Answer from the drawing. Dimensions are ordinates in mm from the lowest x, y and z of the part. A direction names the side the tool comes from. Coordinates: 2 decimals unless noted, no trailing zeros. Order: outer loops, then holes, each group sorted by start corner. A loop starts at its lowest first (then second) coordinate and runs counter-clockwise, first axis right, second up.
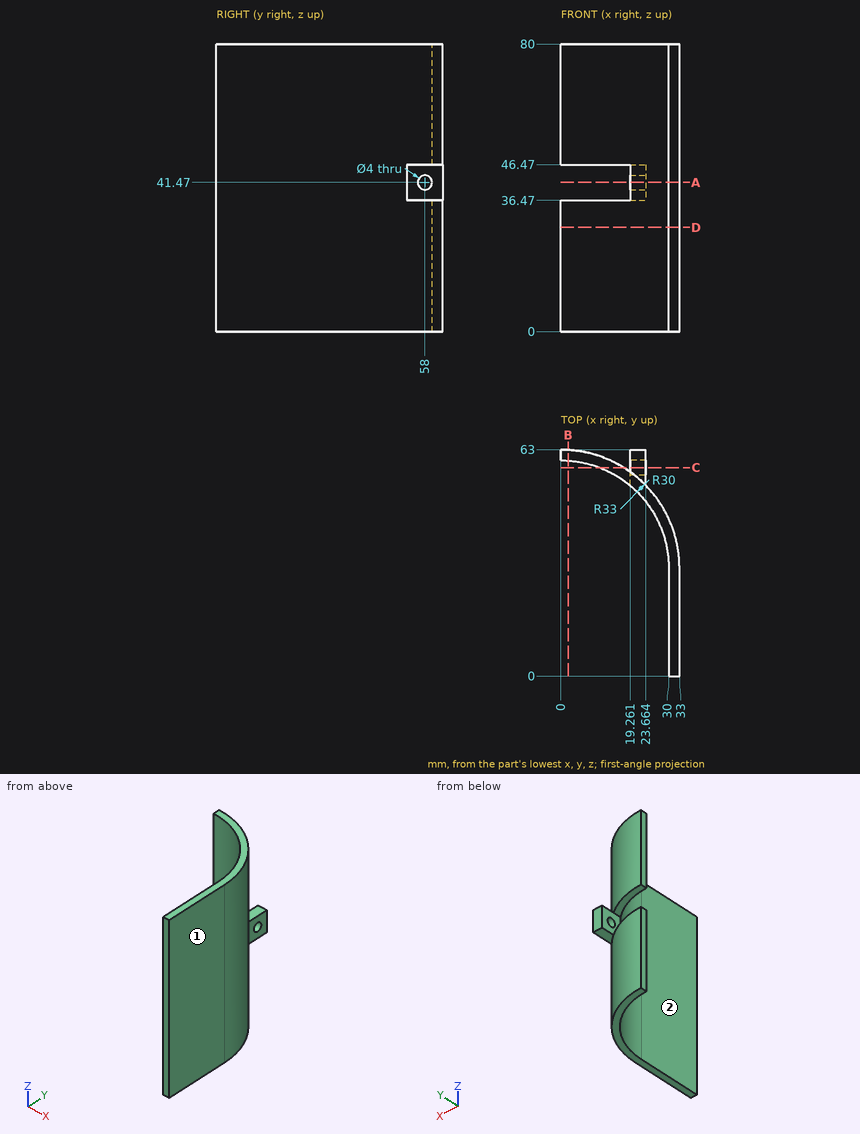
1. Flat-ended cylindrical pins translate along their axes: pin 1 (3 mm diameter, centred on y = 59, z = 39, fed in from -X); pin 2 (2 mm diameter, centred on x = 21, y = 60, fed in from +Z); pin 3 (15 mm diameter, centred on y = 16.5, z = 48, fed in from -X). Find the tip coordinate at first contact, or state that the pin passes through.
2. Consider probe 1 along Z at (x, y) = (21.85, 58); probe 2 along X at (y, z) = (14.5, 27.5); probe 3 along Y at (x, z) = (20, 41) (1 decimal). Determine where each line is inside the solid, lowest interval first.
3. The part is cut by section C-C (y = 58). Determine the outline of the cut face in (x, z) (1 decimal), plus the area to 3 significant figures.
4. The part is cut by section D-D (z = 29). Determine the outline of the cut face in (x, y).
5. The part is cut by section A-A (z = 41.47). Determine the outline of the cut face in (x, y) (1 decimal), plus the area to 3 significant figures.
6. For the marked faces 1 and 2, determine the directions among +Z, -Z, +X, -X, +Y, -Y from which every point of the face is accessible in a straight line to the end or side of a thin tool.
7. The part is cut by section B-B (x = 2). Determine the outline of the cut face in (y, z).
Worked out:
1. pin 1: stops at x = 19.26
1. pin 2: stops at z = 46.47
1. pin 3: stops at x = 30
2. probe 1: z = 36.47 to 39.47, 43.47 to 46.47
2. probe 2: x = 30 to 33
2. probe 3: y = 52.4 to 56.1, 59.9 to 63
3. outline: (10.8, 0) - (17.5, 0) - (17.5, 36.5) - (10.8, 36.5) - close; (10.8, 46.5) - (17.5, 46.5) - (17.5, 80) - (10.8, 80) - close; (19.3, 36.5) - (23.7, 36.5) - (23.7, 39.5) - (19.3, 39.5) - close; (19.3, 43.5) - (23.7, 43.5) - (23.7, 46.5) - (19.3, 46.5) - close
3. area: 495 mm2
4. outline: (0, 60) arc R30 cw to (30, 30) - (30, 0) - (33, 0) - (33, 30) arc R33 ccw to (0, 63) - close
5. outline: (19.3, 53) arc R30 cw to (30, 30) - (30, 0) - (33, 0) - (33, 30) arc R33 ccw to (23.7, 53) - (23.7, 56) - (19.3, 56) - close; (19.3, 60) - (23.7, 60) - (23.7, 63) - (19.3, 63) - close
5. area: 194 mm2
6. face 1: +Z, -Z, +X, +Y, -Y
6. face 2: +Z, -Z, -X, -Y
7. outline: (59.93, 0) - (62.94, 0) - (62.94, 36.47) - (59.93, 36.47) - close; (59.93, 46.47) - (62.94, 46.47) - (62.94, 80) - (59.93, 80) - close
